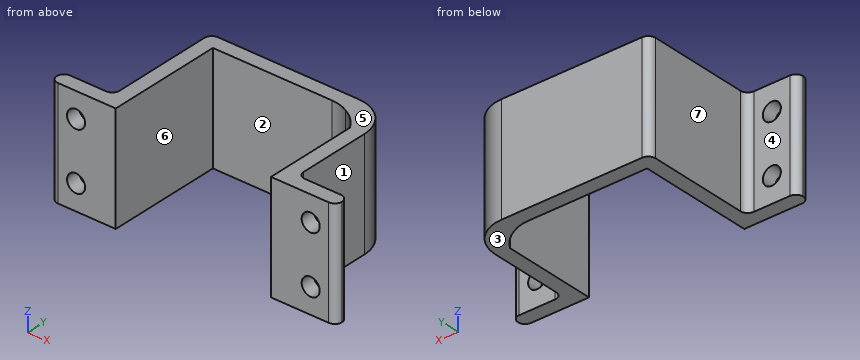
```python
from build123d import *

# Parameters (mm, degrees)
BOSS_EXTRUDE1_DEPTH = 30
SKETCH2_R           = 2.5
CUT_EXTRUDE1_DEPTH  = 91.360389552
CUT_EXTRUDE2_DEPTH  = 92.853143659
FILLET1_R           = 2


with BuildPart() as part:
    # Sketch1 → Boss-Extrude1 (new body)
    with BuildSketch(Plane.XY):
        with BuildLine():
            Line((0, 0), (18, 0))
            Line((18, 0), (18, 32))
            Line((18, 32), (51, 32))
            ThreePointArc((51, 32), (58.071067812, 29.071067812), (61, 22))
            Line((61, 22), (61, 0))
            Line((61, 0), (79, 0))
            Line((79, 0), (79, 4))
            Line((79, 4), (65, 4))
            Line((65, 4), (65, 26))
            ThreePointArc((65, 26), (62.071067812, 33.071067812), (55, 36))
            Line((55, 36), (14, 36))
            Line((14, 36), (14, 4))
            Line((14, 4), (0, 4))
            Line((0, 4), (0, 0))
        make_face()
    extrude(amount=BOSS_EXTRUDE1_DEPTH)

    # Sketch2 → Cut-Extrude1 (cut, through all)
    with BuildSketch(Plane(origin=(0, 4, 0), x_dir=(1, 0, 0), z_dir=(0, 1, 0))):
        with Locations(Location((7, -7, 0), (0, 0, 270))):
            Circle(SKETCH2_R)
        with Locations(Location((7, -23, 0), (0, 0, 270))):
            Circle(SKETCH2_R)
        with Locations(Location((72, -7, 0), (0, 0, 270))):
            Circle(SKETCH2_R)
        with Locations(Location((72, -23, 0), (0, 0, 270))):
            Circle(SKETCH2_R)
    extrude(amount=-CUT_EXTRUDE1_DEPTH, mode=Mode.SUBTRACT)

    # Sketch3 → Cut-Extrude2 (cut, through all)
    with BuildSketch(Plane.XY.offset(30)):
        with BuildLine():
            ThreePointArc((55.768474142, 30.789860884), (59.593158366, 27.114452981), (61, 22))
            Line((61, 22), (61, 26.007623502))
            ThreePointArc((61, 26.007623502), (58.735019606, 28.782480547), (55.768474142, 30.789860884))
        make_face()
    extrude(amount=-CUT_EXTRUDE2_DEPTH, mode=Mode.SUBTRACT)

    # Fillet1
    fillet1_edges = [part.edges().sort_by_distance(p)[0] for p in [
        (79, 0, 15),
        (79, 4, 15),
        (65, 4, 15),
        (14, 36, 15),
        (0, 0, 15),
        (0, 4, 15),
        (14, 4, 15),
    ]]
    fillet(fillet1_edges, radius=FILLET1_R - 0.0001)  # a hair under: the kernel refuses the full size


solid = part.part
```
Verification items for the finished model (mm, model axes). Face numbers are marked on the shaded views. A direction names the side the tool comes from. Give positions to 0.01 mm unless a question says otherwise; leave off trailing zeros. Loops run counter-clockwise (first coordinate to the right, second up) from the corner with the lowest first, then second, coordinate; pieces in that order, holes last.
1. Go/stop test with flat-tipped pins: pin 1 Ø4 at (x, z) = (11, 26) entering from +Y; pin 2 Ø5 at (x, z) = (71.5, 11.5) entering from +Y; pin 3 Ø2 at (y, z) = (26, 5) entering from +X. Record where each tip stops, or that it passes through.
2. Thickness scan on line 1 (X direction, y = 16, z = 19.5); line 2 (X direction, y = 1.7, z = 23); line 3 (Y direction, x = 35, z = 12.5). Record the ranges inside material, lowest first.
3. Set-up check for the marked faces 1, 2, 3 and 4: record each of +Z, -Z, +X, -X, +Y, -Y from which the full face is reachable in a straight line by a thin tool's end or side.
4. Section check C-C, the plane y = 30. Enter the section's corners in (x, z).
5. Mould release check, pull along X, two halves, no side actions. Record for the marked faces 5, 6 and 7: released by +X, released by -X, zero draft, split by the parting line, or undercut.
6. Section check B-B, the plane x = 72. Enter the section's corners in (y, z), then the cut area to 3 significant figures.
7. Section check A-A, the plane z = 5.5. Count the separate pieces of the cut face and the enclosed holes in it, then the cut area to 3 significant figures.
Geometry says:
1. pin 1: stops at y = 4.27
1. pin 2: stops at y = 4
1. pin 3: stops at x = 65
2. line 1: x = 14 to 18, 61 to 65
2. line 2: x = 0.02 to 4.5, 9.5 to 18, 61 to 69.5, 74.5 to 78.98
2. line 3: y = 32 to 36
3. face 1: +Z, -Z, +X, +Y
3. face 2: +Z, -Z, -Y
3. face 3: -Z, +X, -X, +Y, -Y
3. face 4: +Z, -Z, -X, +Y
4. outline: (14, 0) - (18, 0) - (18, 30) - (14, 30) - close; (57.17, 0) - (64.17, 0) - (64.17, 30) - (57.17, 30) - close
5. face 5: zero draft
5. face 6: undercut
5. face 7: released by -X
6. outline: (0, 0) - (4, 0) - (4, 4.5) - (0, 4.5) - close; (0, 9.5) - (4, 9.5) - (4, 20.5) - (0, 20.5) - close; (0, 25.5) - (4, 25.5) - (4, 30) - (0, 30) - close
6. area: 80.0 mm2
7. separate pieces: 3
7. enclosed holes: 0
7. area: 534 mm2
